Source: CAD feature listing. Evaluate the final solid. Frame: model axes, mm. A direction names the side the tool comes from. Give positions to 0.01 mm unless a question says otherwise; leave off trailing zeros. Order: outer loops, then holes, each group sorted by start corner. A loop starts at its lowest first (then second) coordinate and runs counter-clockwise, first axis right, second up.
1) Access query for faces 1 (the face through (-352.291, -15, 164)), 2 (the face through (-282.13, 0.99, 157.48)), 3 (the face through (-294, 2, 167)). Directions: +Z, -Z, +X, -X, +Y, -Y. A direction counts if a zero-diameter tool reaches every point of the face in a straight line with its end or side. Return the directions, or none.
2) Material intervals for line 1 (X direction, y = -18.25, z = 15); line 2 (Z direction, x = 4, y = -24.5); line 3 (Y direction, x = -128.5, z = 25), sorted ascending.
3) Section D-D, the plane x = -303. Return loops of the section in (y, z), plus the area to 3 significant figures.
4) Draft query along X for faces 4 (the face through (-354.291, -14, 164)), 5 (the face through (-157, -14, -33.396)), 6 (the face through (-157, -2, 169)), 7 (the face through (45.709, -14, 164)). Return one class per face: released by +X, released by -X, zero draft, split by the parting line, or undercut.
5) Section A-A, the plane y = -17.25. Return loops of the section in (x, z).
6) Section C-C, the plane z = 317.5. Return loops of the section in (x, y), plus the area to 3 significant figures.
7) First-contact query: P1, Ø3, axis at x = -101.5, z = 51, coming from the +Y side; P2, Ø1, axis at x = -4.5, z = 11.5, coming from the -Y side. Flat tips, straight axial feed; report the tip coordinate or a pass-through.
8) Section B-B, the plane x = 16. Return loops of the section in (y, z), plus the area to 3 significant figures.
```python
from build123d import *

# Parameters (mm, degrees)
F0_W     = 400
F0_H     = 400
F1_DEPTH = 28
F2_W     = 396
F2_H     = 396
F3_DEPTH = 26
F4_R     = 15
F5_DEPTH = 2


with BuildPart() as f1:
    # F0 (on Front) → F1 (new body)
    with BuildSketch(Plane.XZ):
        with Locations((-154.291336, 166.60433)):
            Rectangle(F0_W, F0_H)
    extrude(amount=F1_DEPTH)

    # F2 (on face) → F3 (cut)
    with BuildSketch(Plane.XZ.offset(28)):
        with Locations((-154.291336, 166.60433)):
            Rectangle(F2_W, F2_H)
    extrude(amount=-F3_DEPTH, mode=Mode.SUBTRACT)

    # F4 (on face) → F5 (join)
    with BuildSketch(Plane(origin=(0, 0, 0), x_dir=(-1, 0, 0), z_dir=(0, 1, 0))):
        with Locations((294.033349, 166.60433)):
            Circle(F4_R)
    extrude(amount=F5_DEPTH)


solid = f1.part
```
From the geometry:
1. face 1: -Y
1. face 2: +Y
1. face 3: +Z, -Z, +X, -X, +Y
2. line 1: x = -354.29 to -352.29, 43.71 to 45.71
2. line 2: z = -33.4 to -31.4, 364.6 to 366.6
2. line 3: y = -2 to 0
3. outline: (-28, -33.4) - (0, -33.4) - (0, 154.58) - (2, 154.58) - (2, 178.63) - (0, 178.63) - (0, 366.6) - (-28, 366.6) - (-28, 364.6) - (-2, 364.6) - (-2, -31.4) - (-28, -31.4) - close
3. area: 952 mm2
4. face 4: released by -X
4. face 5: zero draft
4. face 6: undercut
4. face 7: released by +X
5. outline: (-354.29, -33.4) - (45.71, -33.4) - (45.71, 366.6) - (-354.29, 366.6) - close; hole (-352.29, -31.4) - (43.71, -31.4) - (43.71, 364.6) - (-352.29, 364.6) - close
6. outline: (-354.29, -28) - (-352.29, -28) - (-352.29, -2) - (43.71, -2) - (43.71, -28) - (45.71, -28) - (45.71, 0) - (-354.29, 0) - close
6. area: 904 mm2
7. P1: stops at y = 0
7. P2: stops at y = -2
8. outline: (-28, -33.4) - (0, -33.4) - (0, 366.6) - (-28, 366.6) - (-28, 364.6) - (-2, 364.6) - (-2, -31.4) - (-28, -31.4) - close
8. area: 904 mm2
